Study the drawing (mm; zero at the part's minimum x, y, z) and answer. A direction names the side the tool comes from. Coordinates: 2 decimals unless noted, no trailing zeros. Order: outer loops, then holes, each group sorted by start corner. A loop starts at its lowest first (then second) coordinate and runs counter-clockwise, first axis right, second up.
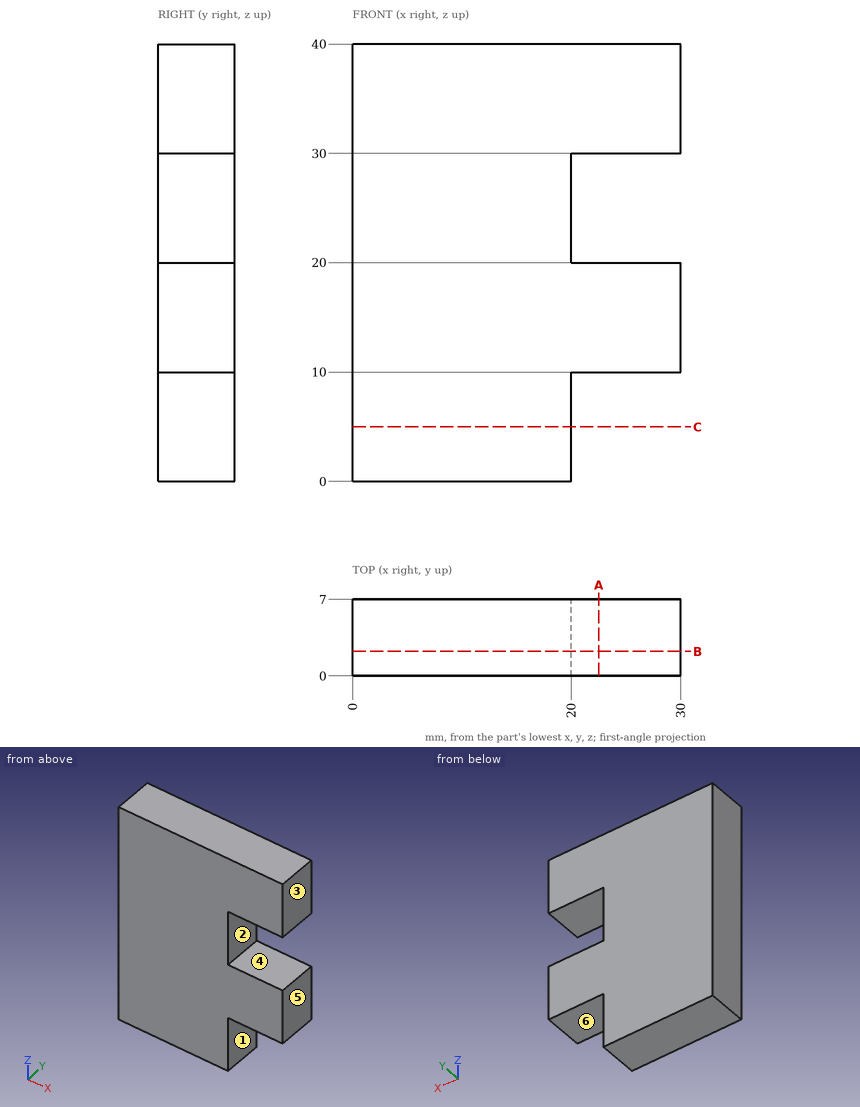
(1) Consider line 1 (Z direction, x = 21.75, y = 2); line 2 (X direction, y = 5.75, z = 21.5). Determine where each line is inside the solid, lowest interval first.
(2) The mould has two halves that part along Z. Classify the marked faces 4, 5 and 6: released by +Z, released by -Z, zero draft, split by the parting line, or undercut.
(3) Find section C-C (z = 5). Write down the section's boundary in (x, y), and give its area (3 significant figures).
(4) Find section B-B (y = 2.25). Write down the section's boundary in (x, z), and give its area (3 significant figures).
(5) Find section A-A (x = 22.5). Write down the section's boundary in (y, z).
(6) Each of these flat-tipped pins is pushed along its axis until it touches: pin 1 Ø2 at (x, y) = (25, 2) entering from -Z; pin 2 Ø2 at (y, z) = (5, 4.5) entering from +X. Where does it stop, or does it pass through?
(7) For the marked faces 1, 2 and 3, determine the directions among +Z, -Z, +X, -X, +Y, -Y from which every point of the face is accessible in a straight line to the end or side of a thin tool.
Findings below:
1. line 1: z = 10 to 20, 30 to 40
1. line 2: x = 0 to 20
2. face 4: undercut
2. face 5: zero draft
2. face 6: released by -Z
3. outline: (0, 0) - (20, 0) - (20, 7) - (0, 7) - close
3. area: 140 mm2
4. outline: (0, 0) - (20, 0) - (20, 10) - (30, 10) - (30, 20) - (20, 20) - (20, 30) - (30, 30) - (30, 40) - (0, 40) - close
4. area: 1,000 mm2
5. outline: (0, 10) - (7, 10) - (7, 20) - (0, 20) - close; (0, 30) - (7, 30) - (7, 40) - (0, 40) - close
6. pin 1: stops at z = 10
6. pin 2: stops at x = 20
7. face 1: -Z, +X, +Y, -Y
7. face 2: +X, +Y, -Y
7. face 3: +Z, -Z, +X, +Y, -Y
